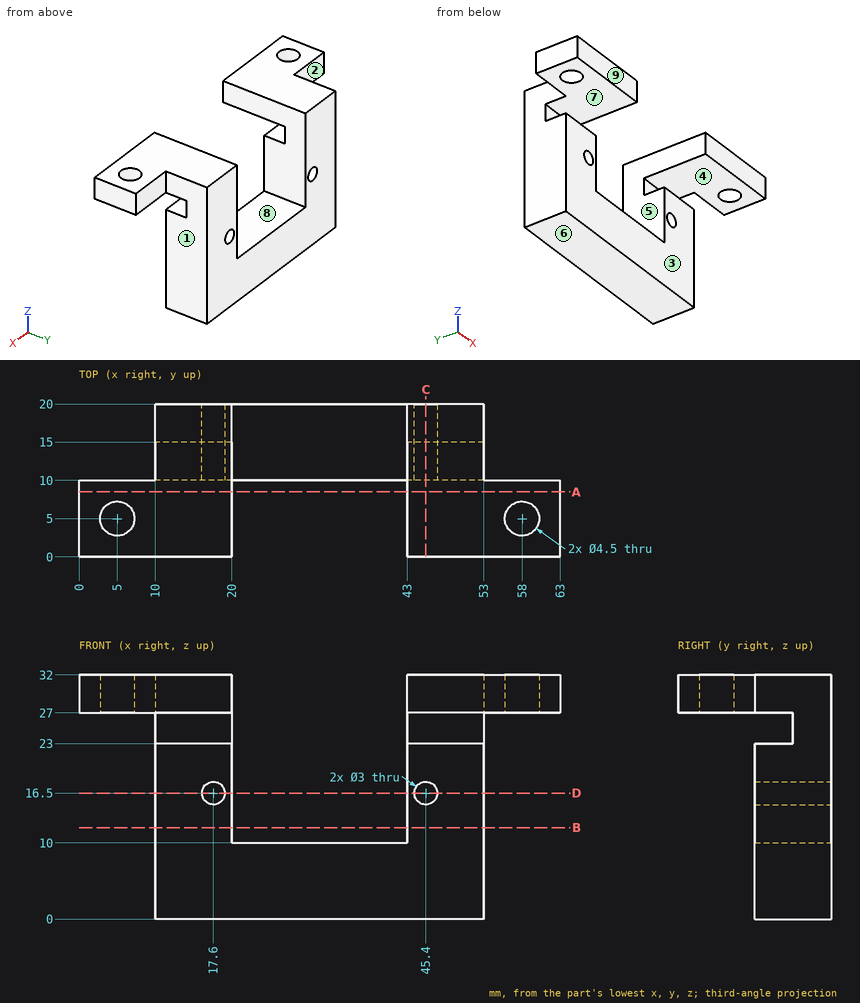
Geometry: see drawing. Coordinates: mm, zero at the bounding-box minimum. A direction names the side the tool comes from. Coordinates: 2 decimals unless noted, no trailing zeros. Order: outer loops, then holes, each group sorted by start corner. A loop starts at its lowest first (then second) coordinate and runs counter-clockwise, first axis right, second up. Notation, with made-up numbers: M 15.25,27 L 73.25,27 A17 cw 73.25,33 Z; hole C 73,23.5 d1. An arc over 180 degrees is marked long. Answer as CSV lines item,"result".
1. Material intervals for line 1 (X direction, y = 14.5, z = 16.5); line 2 (X direction, y = 4.5, z = 28); line 3 (X direction, y = 19.25, z = 19), sorted ascending. Write a range as from..to.
Reported:
line 1,"10..16.1, 19.1..20, 43..43.9, 46.9..53"
line 2,"0..2.81, 7.19..20, 43..55.81, 60.19..63"
line 3,"10..20, 43..53"
2. Access query for the marked faces 1, 2, 3, 4 and 5. Directions: +Z, -Z, +X, -X, +Y, -Y. A direction counts if a zero-diameter tool reaches every point of the face in a straight line with its end or side. Return the directions, or none.
Reported:
face 1,"+Z, -Z, +X, +Y"
face 2,"+Z, -Z, -X, +Y"
face 3,"-Z, +X, -X, -Y"
face 4,"+X, -X, -Y"
face 5,"+Z, +Y, -Y"
3. Section A-A (y = 8.5). Return the cut outline in (x, z).
Reported:
outline,"M 0,27 L 20,27 L 20,32 L 0,32 Z; M 43,27 L 63,27 L 63,32 L 43,32 Z"
4. Section B-B (z = 12). Return the cut outline in (x, y).
Reported:
outline,"M 10,10 L 20,10 L 20,20 L 10,20 Z; M 43,10 L 53,10 L 53,20 L 43,20 Z"
5. Pull-direction query (Z, two-part tool) for the marked faces 6, 7, 8 and 9; classes: released by +Z, released by -Z, zero draft, split by the parting line, or undercut.
Reported:
face 6,"released by -Z"
face 7,"undercut"
face 8,"released by +Z"
face 9,"zero draft"
6. First-contact query: P1, Ø1.5, axis at x = 28, z = 12.5, coming from the +Y side; P2, Ø3, axis at x = 29, y = 12.5, coming from the +Z side; P3, Ø5, axis at x = 58, y = 5, coming from the -Z side; P4, Ø3, axis at y = 14.5, z = 8.5, coming from the +X side. Flat tips, straight axial feed; report the tip coordinate or a pass-through.
Reported:
P1,"through"
P2,"z = 10"
P3,"z = 27"
P4,"x = 53"
7. Section C-C (x = 45.4). Return the cut outline in (y, z).
Reported:
outline,"M 0,27 L 15,27 L 15,23 L 10,23 L 10,18 L 20,18 L 20,32 L 0,32 Z; M 10,0 L 20,0 L 20,15 L 10,15 Z"
8. Section D-D (z = 16.5). Return the cut outline in (x, y), then the cut area to 3 significant figures.
Reported:
outline,"M 10,10 L 16.1,10 L 16.1,20 L 10,20 Z; M 19.1,10 L 20,10 L 20,20 L 19.1,20 Z; M 43,10 L 43.9,10 L 43.9,20 L 43,20 Z; M 46.9,10 L 53,10 L 53,20 L 46.9,20 Z"
area,"140 mm2"
